```python
from build123d import *

# Parameters (mm, degrees)
F0_W          = 50
F0_H          = 50
F1_DEPTH      = 25
F1_DEPTH_BACK = 25
F2_R          = 4
F3_DEPTH      = 25
F4_SIZE       = 7
F5_R          = 5
F6_R          = 2.5
F7_DEPTH      = 50


with BuildPart() as f1:
    # F0 (on Front) → F1 (new body, two sides)
    with BuildSketch(Plane.XZ) as f1_sk:
        Rectangle(F0_W, F0_H)
    extrude(amount=F1_DEPTH)
    extrude(f1_sk.sketch, amount=-F1_DEPTH_BACK)

    # F2 (on face) → F3 (join)
    with BuildSketch(Plane.XZ.offset(25)):
        Circle(F2_R)
    extrude(amount=F3_DEPTH)

    # F4
    f4_edges = [f1.edges().sort_by_distance(p)[0] for p in [
        (-25, 0, 25),
        (25, 0, 25),
        (25, 0, -25),
        (-25, 0, -25),
    ]]
    chamfer(f4_edges, length=F4_SIZE)

    # F5
    f5_edges = [f1.edges().sort_by_distance(p)[0] for p in [
        (-18, 0, 25),
        (-25, 0, 18),
        (18, 0, 25),
        (25, 0, 18),
        (25, 0, -18),
        (18, 0, -25),
        (-18, 0, -25),
        (-25, 0, -18),
    ]]
    fillet(f5_edges, radius=F5_R)

    # F6 (on face) → F7 (cut)
    with BuildSketch(Plane(origin=(0, 25, 0), x_dir=(-1, 0, 0), z_dir=(0, 1, 0))):
        with Locations((-15, 15)):
            Circle(F6_R)
        with Locations((15, 15)):
            Circle(F6_R)
        with Locations((15, -15)):
            Circle(F6_R)
        with Locations((-15, -15)):
            Circle(F6_R)
    extrude(amount=-F7_DEPTH, mode=Mode.SUBTRACT)


solid = f1.part
```
Geometry check sheet. Reference: the model listing, model coordinates, mm. A direction names the side the tool comes from. Coordinates: 2 decimals unless noted, no trailing zeros. Loops run counter-clockwise (first coordinate to the right, second up) from the corner with the lowest first, then second, coordinate; pieces in that order, holes last. Notation, with made-up numbers: (54.5, 62) - (108.5, 62) arc R19 ccw to (108.5, 87) - close; hole circle Ø2 at (16.5, -2). An arc over 180 degrees is marked (long way). One line per item, written item: value. Start each with the question number.
(1) Cross-section at B-B on y = 17.5. Enter the section's corners in (x, z), plus the area to 3 significant figures.
(2) Cross-section at A-A on z = -15. Enter the section's corners in (x, y).
(3) Material ranges on line 1 (Z direction, x = -15, y = 7); line 2 (X direction, y = 6.5, z = 17); line 3 (X direction, y = 5.5, z = 16.5), recorded low to high. Write a range as [from, to].
(4) Tool access check on faces 1 (the cylindrical face through (-17.87, 0.35, 24.61)), 2 (the cylindrical face through (-0.867, -37.325, -3.905)). Record the directions out of +Z, -Z, +X, -X, +Y, -Y that give a thin tool (end or side, any length) a straight path to the whole face; none if there is none.
(5) Cross-section at D-D on z = 0. Enter the section's corners in (x, y).
(6) Cross-section at C-C on x = -15. Enter the section's corners in (y, z), plus the area to 3 significant figures.
(7) Depth check by flat-ended pin: P1, Ø10, axis at x = 16.5, z = -16, coming from the -Y side; P2, Ø1, axis at x = 18, y = -18, coming from the -Z side. Enter the tip coordinate at first touch or a pass-through.
(8) Mould release check, pull along X, two halves, no side actions. Record for faces 3 (the flat face through (-21, 0, 22)), 4 (the flat face through (0, 0, -25)), 5 (the cylindrical face through (-12.5, 0.4, -14.9)): released by +X, released by -X, zero draft, split by the parting line, or undercut.
Results below:
1. outline: (-25, -15.93) arc R5 ccw to (-23.54, -19.46) - (-19.46, -23.54) arc R5 ccw to (-15.93, -25) - (15.93, -25) arc R5 ccw to (19.46, -23.54) - (23.54, -19.46) arc R5 ccw to (25, -15.93) - (25, 15.93) arc R5 ccw to (23.54, 19.46) - (19.46, 23.54) arc R5 ccw to (15.93, 25) - (-15.93, 25) arc R5 ccw to (-19.46, 23.54) - (-23.54, 19.46) arc R5 ccw to (-25, 15.93) - close; hole circle Ø5 at (-15, -15); hole circle Ø5 at (-15, 15); hole circle Ø5 at (15, -15); hole circle Ø5 at (15, 15)
1. area: 2,320 mm2
2. outline: (-25, -25) - (-17.5, -25) - (-17.5, 25) - (-25, 25) - close; (-12.5, -25) - (12.5, -25) - (12.5, 25) - (-12.5, 25) - close; (17.5, -25) - (25, -25) - (25, 25) - (17.5, 25) - close
3. line 1: z = [-25, -17.5], [-12.5, 12.5], [17.5, 25]
3. line 2: x = [-24.88, -16.5], [-13.5, 13.5], [16.5, 24.88]
3. line 3: x = [-24.97, -17], [-13, 13], [17, 24.97]
4. face 1: +Z, -X, +Y, -Y
4. face 2: -Y
5. outline: (-25, -25) - (-4, -25) - (-4, -50) - (4, -50) - (4, -25) - (25, -25) - (25, 25) - (-25, 25) - close
6. outline: (-25, -25) - (25, -25) - (25, -17.5) - (-25, -17.5) - close; (-25, -12.5) - (25, -12.5) - (25, 12.5) - (-25, 12.5) - close; (-25, 17.5) - (25, 17.5) - (25, 25) - (-25, 25) - close
6. area: 2,000 mm2
7. P1: stops at y = -25
7. P2: stops at z = -24.75
8. face 3: released by -X
8. face 4: zero draft
8. face 5: undercut
